Check sheet for the modelled part. Datum: model origin and axes. Units: mm. A direction names the side the tool comes from. Give positions to 0.01 mm unless a question says otherwise; leave off trailing zeros. Write each loop counter-clockwise with the first axis right and the second up, starting at its lowest first coordinate (ties: lowest second). Pieces come first, ordered by that corner, then holes. Notation, with made-up numbers: M 68,-30 L 105,-30 A30 ccw 105,7 Z; hole C -0.5,74.5 d6. An arc over 180 degrees is marked long. Write item = value, one per line. Start each with the question number.
1) Set-up check for faces 1 (the face through (4.235, 1.479, 0.364)), 2 (the face through (0.9, 5.96, 2.86)): record each of +Z, -Z, +X, -X, +Y, -Y from which the full face is reachable in a straight line by a thin tool's end or side.
2) Sectioned sample at A-A, the plane y = 1.5. Record the cut outline in (x, z), then the cut area to 3 significant figures.
3) Draft check along Z on faces 3 (the face through (-4.235, 1.479, -0.364)), 4 (the face through (2.4, 9, 2.1)), 5 (the face through (-9.76, 7.99, -2.17)). Enter one of: pulls with the +Z half, pulls with the -Z half, needs draft (parallel to the pull), parting line crosses it, or undercut.
4) Gauge pin test, flat ends, axial feed: pin 1 (9 mm diameter, centred on x = 0, z = 0, fed in from -Y); pin 2 (3 mm diameter, centred on x = 3, y = 6, fed in from -Z); pin 3 (8 mm diameter, centred on x = 0, z = 0, fed in from -Y); pin 4 (3 mm diameter, centred on y = 8, z = 4.5, fed in from -X). Record the tip position at first contact, or that the pin passes through.
5) Scan lines: L1, parallel to X at y = 6, z = 0; L2, parallel to Z at x = 0.5, y = 0.5; L3, parallel to Z at x = 0, y = 6.9. Record each from-to range of solid material in increasing order.
6) Sectioned sample at B-B, the plane y = 3.25. Record the cut outline in (x, z), then the cut area to 3 significant figures.
from build123d import *

# Parameters (mm, degrees)
SKETCH1_R           = 7
SKETCH1_R_2         = 3
BOSS_EXTRUDE1_DEPTH = 9
BOSS_EXTRUDE2_START = -3
SKETCH2_R           = 10
SKETCH2_R_2         = 3
BOSS_EXTRUDE2_DEPTH = 3
CUT_EXTRUDE1_DEPTH  = 3
CHAMFER1_SIZE       = 2
CHAMFER2_SIZE       = 1
FILLET1_R           = 1


with BuildPart() as part:
    # Sketch1 → Boss-Extrude1 (new body)
    with BuildSketch(Plane(origin=(0, 0, 0), x_dir=(1, 0, 0), z_dir=(0, 1, 0))):
        with Locations(Location((0, 0, 0), (0, 0, 270))):
            Circle(SKETCH1_R)
        with Locations(Location((0, 0, 0), (0, 0, 270))):
            Circle(SKETCH1_R_2, mode=Mode.SUBTRACT)
    extrude(amount=BOSS_EXTRUDE1_DEPTH)

    # Sketch2 → Boss-Extrude2 (add)
    with BuildSketch(Plane(origin=(0, 9, 0), x_dir=(1, 0, 0), z_dir=(0, 1, 0)).offset(BOSS_EXTRUDE2_START)):
        with Locations(Location((0, 0, 0), (0, 0, 270))):
            Circle(SKETCH2_R)
        with Locations(Location((0, 0, 0), (0, 0, 270))):
            Circle(SKETCH2_R_2, mode=Mode.SUBTRACT)
    extrude(amount=BOSS_EXTRUDE2_DEPTH)

    # Sketch3 → Cut-Extrude1 (cut)
    with BuildSketch(Plane.XZ):
        Polygon((-4.001709946, -2.840713087), (0.459274725, -4.885939015), (4.460984671, -2.045225929), (4.001709946, 2.840713087), (-0.459274725, 4.885939015), (-4.460984671, 2.045225929), align=None)
    extrude(amount=-CUT_EXTRUDE1_DEPTH, mode=Mode.SUBTRACT)

    # Chamfer1
    chamfer1_edges = [part.edges().sort_by_distance(p)[0] for p in [
        (0, 6, -7),
    ]]
    chamfer(chamfer1_edges, length=CHAMFER1_SIZE)

    # Chamfer2
    chamfer2_edges = [part.edges().sort_by_distance(p)[0] for p in [
        (0, 6, -10),
    ]]
    chamfer(chamfer2_edges, length=CHAMFER2_SIZE - 0.0001)  # a hair under: the kernel refuses the full size

    # Fillet1
    fillet1_edges = [part.edges().sort_by_distance(p)[0] for p in [
        (0, 4, -7),
    ]]
    fillet(fillet1_edges, radius=FILLET1_R)


solid = part.part
Data:
q1.face_1 = -Y
q1.face_2 = +Y, -Y
q2.outline = C 0,0 d14; hole M -4.46,2.05 L -4,-2.84 L 0.46,-4.89 L 4.46,-2.05 L 4,2.84 L -0.46,4.89 Z
q2.area = 91.4 mm2
q3.face_3 = undercut
q3.face_4 = needs draft
q3.face_5 = parting line crosses it
q4.pin_1 = 0
q4.pin_2 = -9.82
q4.pin_3 = 3
q4.pin_4 = -9.54
q5.L1 = -9 to -3, 3 to 9
q5.L2 = -6.98 to -4.86, 4.45 to 6.98
q5.L3 = -9.9 to -3, 3 to 9.9
q6.outline = C 0,0 d14; hole C 0,0 d6
q6.area = 126 mm2
